Check sheet for the modelled part. Datum: model origin and axes. Units: mm. Round coordinates to 2 decimals unless told otherwise and drop trailing zeros. Order: outer loops, then holes, each group sorted by start corner. A loop starts at its lowest first (then second) coordinate and runs counter-clockwise, first axis right, second up.
Q1. Cross-section at D-D on x = 33.02. Record the cut outline in (y, z) (3 decimals), then the cut area to 3 significant figures.
Q2. Cross-section at C-C on y = 2.25. Record the cut outline in (x, z), then the cut area to 3 significant figures.
Q3. Cross-section at A-A on z = 0. Record the cut outline in (x, y) (3 decimals).
Q4. Depth check by flat-ended pin: P1, Ø1, axis at y = 2.5, z = 31.5, coming from the +X side. Enter the tip coordinate at first touch or a pass-through.
Q5. Cross-section at B-B on x = 11.5. Record the cut outline in (y, z) (3 decimals).
Q6. Scan lines: probe 1 along X at (y, z) = (0.2, -41); probe 2 along Z at (x, y) = (33.02, 1.1); probe 3 along X at (y, z) = (3.05, -5.5). Record each from-to range of solid material in increasing order.
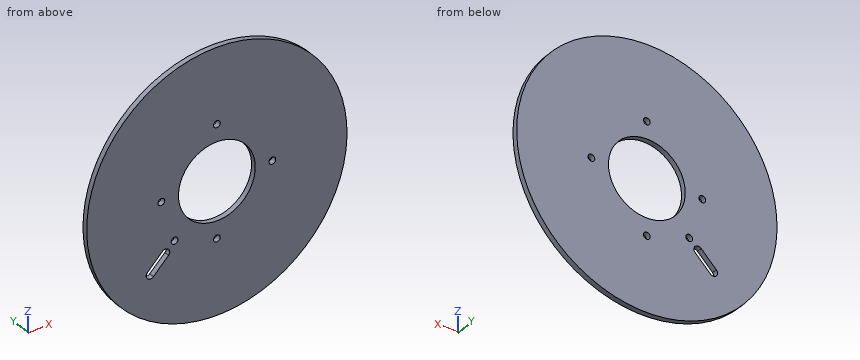
from build123d import *

# Parameters (mm, degrees)
SKETCH1_R           = 77.4600051
BOSS_EXTRUDE1_DEPTH = 3.175
SKETCH20_R          = 22.86
SKETCH20_R_2        = 2.0193
CUT_EXTRUDE10_DEPTH = 250.596695835
CUT_EXTRUDE11_DEPTH = 3.175
SKETCH22_R          = 2.0193
CUT_EXTRUDE12_DEPTH = 250.596695835


with BuildPart() as part:
    # Sketch1 → Boss-Extrude1 (new body)
    with BuildSketch(Plane(origin=(0, 0, 0), x_dir=(1, 0, 0), z_dir=(0, 1, 0))):
        with Locations(Location((0, 0, 0), (0, 0, 270))):
            Circle(SKETCH1_R)
    extrude(amount=BOSS_EXTRUDE1_DEPTH)

    # Sketch20 → Cut-Extrude10 (cut, through all)
    with BuildSketch(Plane(origin=(-73.768816189, 3.175, -121.080352405), x_dir=(1, 0, 0), z_dir=(0, 1, 0))):
        with Locations(Location((73.768816189, -121.080352405, 0), (0, 0, 270))):
            Circle(SKETCH20_R)
        with Locations(Location((73.768816189, -88.060352405, 0), (0, 0, 270))):
            Circle(SKETCH20_R_2)
        with Locations(Location((106.788816189, -121.080352405, 0), (0, 0, 270))):
            Circle(SKETCH20_R_2)
        with Locations(Location((73.768816189, -154.100352405, 0), (0, 0, 270))):
            Circle(SKETCH20_R_2)
        with Locations(Location((40.748816189, -121.080352405, 0), (0, 0, 270))):
            Circle(SKETCH20_R_2)
    extrude(amount=-CUT_EXTRUDE10_DEPTH, mode=Mode.SUBTRACT)

    # Sketch21 → Cut-Extrude11 (cut)
    with BuildSketch(Plane(origin=(-73.768816189, 3.175, -121.080352405), x_dir=(1, 0, 0), z_dir=(0, 1, 0))):
        with BuildLine():
            Line((41.420818538, -92.324457203), (32.440562417, -83.344201082))
            ThreePointArc((32.440562417, -83.344201082), (32.440562417, -79.752098633), (36.032664865, -79.752098633))
            Line((36.032664865, -79.752098633), (45.012920986, -88.732354754))
            ThreePointArc((45.012920986, -88.732354754), (45.012920986, -92.324457203), (41.420818538, -92.324457203))
        make_face()
    extrude(amount=-CUT_EXTRUDE11_DEPTH, mode=Mode.SUBTRACT)

    # Sketch22 → Cut-Extrude12 (cut, through all)
    with BuildSketch(Plane(origin=(-73.768816189, 3.175, -121.080352405), x_dir=(1, 0, 0), z_dir=(0, 1, 0))):
        with Locations(Location((48.605023435, -95.916559651, 0), (0, 0, 270))):
            Circle(SKETCH22_R)
    extrude(amount=-CUT_EXTRUDE12_DEPTH, mode=Mode.SUBTRACT)


solid = part.part
Results found:
1. outline: (0, -70.069) - (3.175, -70.069) - (3.175, -2.019) - (0, -2.019) - close; (0, 2.019) - (3.175, 2.019) - (3.175, 70.069) - (0, 70.069) - close
1. area: 432 mm2
2. outline: circle Ø154.92 at (0, 0); hole (-41.33, -37.74) arc R2.54 ccw to (-37.74, -41.33) - (-28.76, -32.35) arc R2.54 ccw to (-32.35, -28.76) - close; hole circle Ø4.04 at (-33.02, 0); hole circle Ø4.04 at (-25.16, -25.16); hole circle Ø45.72 at (0, 0); hole circle Ø4.04 at (0, -33.02); hole circle Ø4.04 at (0, 33.02); hole circle Ø4.04 at (33.02, 0)
2. area: 17,100 mm2
3. outline: (-77.46, 0) - (-35.039, 0) - (-35.039, 3.175) - (-77.46, 3.175) - close; (-31.001, 0) - (-22.86, 0) - (-22.86, 3.175) - (-31.001, 3.175) - close; (22.86, 0) - (31.001, 0) - (31.001, 3.175) - (22.86, 3.175) - close; (35.039, 0) - (77.46, 0) - (77.46, 3.175) - (35.039, 3.175) - close
4. P1: stops at x = 70.99
5. outline: (0, -76.602) - (3.175, -76.602) - (3.175, -19.757) - (0, -19.757) - close; (0, 19.757) - (3.175, 19.757) - (3.175, 76.602) - (0, 76.602) - close
6. probe 1: x = -65.72 to -41.61, -37.41 to 65.72
6. probe 2: z = -70.07 to -2.02, 2.02 to 70.07
6. probe 3: x = -77.26 to -22.19, 22.19 to 77.26
